from build123d import *

# Parameters (mm, degrees)
F0_W     = 100
F0_H     = 50
F1_DEPTH = 50
F2_R     = 14
F2_R_2   = 12
F3_DEPTH = 25
F4_R     = 10
F5_DEPTH = 90


with BuildPart() as f1:
    # F0 (on Front) → F1 (new body)
    with BuildSketch(Plane.XZ):
        with Locations((55.64848, -2.676977)):
            Rectangle(F0_W, F0_H)
    extrude(amount=F1_DEPTH)

    # F2 (on face) → F3 (join)
    with BuildSketch(Plane(origin=(5.64848, 0, 0), x_dir=(0, -1, 0), z_dir=(-1, 0, 0))):
        with Locations((25, -2.676977)):
            Circle(F2_R)
        with Locations((25, -2.676977)):
            Circle(F2_R_2, mode=Mode.SUBTRACT)
    extrude(amount=F3_DEPTH)

    # F4 (on face) → F5 (cut)
    with BuildSketch(Plane.YZ.offset(105.64848)):
        with Locations((-25, -2.676977)):
            Circle(F4_R)
    extrude(amount=-F5_DEPTH, mode=Mode.SUBTRACT)


solid = f1.part
The listing builds one solid part. Answer for the finished solid, in the listing's coordinates (mm). A direction names the side the tool comes from. Round coordinates to 2 decimals unless told otherwise and drop trailing zeros. Loops run counter-clockwise (first coordinate to the right, second up) from the corner with the lowest first, then second, coordinate; pieces in that order, holes last. Notation, with made-up numbers: M 47,68 L 96,68 A34 ccw 96,101 Z; hole C 10,-40 d8. An arc over 180 degrees is marked long. Write each question's results on one line, items separated by ' | '. Start each with the question number.
1) Which of the six approach directions +Z, -Z, +X, -X, +Y, -Y give full straight-line access (tool end or side, diameter ignored) to faces 4 (the flat face through (5.648, -36, -14)), 5 (the flat face through (-19.352, -19, 8)), 6 (the cylindrical face through (61.278, -15.462, 0.327))?
2) Straight lines are drawn through the part: probe 1 along Z at (x, y) = (100.5, -25); probe 2 along X at (y, z) = (-20.5, -4.5); probe 3 along Z at (x, y) = (80.5, -28.5). For each, find the intervals that lie inside material, in ascending order.
3) Each of these flat-tipped pins is pushed along its axis until it touches: pin 1 (1.5 mm diameter, centred on y = -43.5, z = -4, fed in from -X); pin 2 (1 mm diameter, centred on y = -26.5, z = 6.5, fed in from +X). Where does it stop, or does it pass through?
4) Find section B-B on y = -25. Write down the section's boundary in (x, z).
5) Find section C-C on z = 4.5. Write down the section's boundary in (x, y), plus the area to 3 significant figures.
6) Determine the mould class of faces 1 (the flat face through (55, -25, 22.323)), 2 (the flat face through (5.648, -25, -3)), 3 (the flat face through (55, -25, -27.677)) for opening direction Z: pulls with the +Z half, pulls with the -Z half, needs draft (parallel to the pull), parting line crosses it, or undercut.
7) Find section D-D on y = -3.5. Write down the section's boundary in (x, z), plus the area to 3 significant figures.
8) Find section A-A on x = 26. Write down the section's boundary in (y, z).
Final values:
1) face 4: -X | face 5: +Z, -Z, -X, +Y, -Y | face 6: +X
2) probe 1: -27.68 to -12.68, 7.32 to 22.32 | probe 2: 5.65 to 15.65 | probe 3: -27.68 to -12.04, 6.69 to 22.32
3) pin 1: x = 5.65 | pin 2: x = 15.65
4) outline: M -19.35,-16.68 L 5.65,-16.68 L 5.65,-27.68 L 105.65,-27.68 L 105.65,-12.68 L 15.65,-12.68 L 15.65,7.32 L 105.65,7.32 L 105.65,22.32 L 5.65,22.32 L 5.65,11.32 L -19.35,11.32 L -19.35,9.32 L 5.65,9.32 L 5.65,-14.68 L -19.35,-14.68 Z
5) outline: M -19.35,-37.02 L 5.65,-37.02 L 5.65,-50 L 105.65,-50 L 105.65,-31.96 L 15.65,-31.96 L 15.65,-18.04 L 105.65,-18.04 L 105.65,0 L 5.65,0 L 5.65,-12.98 L -19.35,-12.98 L -19.35,-15.38 L 5.65,-15.38 L 5.65,-34.62 L -19.35,-34.62 Z | area: 3,870 mm²
6) face 1: pulls with the +Z half | face 2: undercut | face 3: pulls with the -Z half
7) outline: M 5.65,-27.68 L 105.65,-27.68 L 105.65,22.32 L 5.65,22.32 Z | area: 5,000 mm²
8) outline: M -50,-27.68 L 0,-27.68 L 0,22.32 L -50,22.32 Z; hole C -25,-2.68 d20
